from build123d import *

# Parameters (mm, degrees)
F0_W     = 33
F0_H     = 5.5
F1_DEPTH = 2
F2_W     = 33
F2_H     = 2
F3_DEPTH = 33
F4_R     = 3
F5_DEPTH = 2.001


with BuildPart() as f1:
    # F0 (on Top) → F1 (new body)
    with BuildSketch(Plane.XY):
        Rectangle(F0_W, F0_H)
    extrude(amount=F1_DEPTH)

    # F2 (on face) → F3 (join)
    with BuildSketch(Plane.XY.offset(2)):
        with Locations((0, 1.75)):
            Rectangle(F2_W, F2_H)
    extrude(amount=F3_DEPTH)

    # F4 (on face) → F5 (cut, through all)
    with BuildSketch(Plane.XZ.offset(-0.75)):
        with Locations((-9, 17)):
            Circle(F4_R)
        with Locations((9, 17)):
            Circle(F4_R)
    extrude(amount=-F5_DEPTH, mode=Mode.SUBTRACT)


solid = f1.part
Can you work these out from the model? Positions are in its coordinate system, mm. A direction names the side the tool comes from. Round coordinates to 2 decimals unless told otherwise and drop trailing zeros. Write each loop counter-clockwise with the first axis right and the second up, starting at its lowest first coordinate (ties: lowest second). Pieces come first, ordered by that corner, then holes. Notation, with made-up numbers: M -17.75,-36.5 L 40.25,-36.5 A23 cw 40.25,-9.5 Z; hole C 23,-35 d10. An arc over 180 degrees is marked long. Use a Markdown table: item, result.
Item 1: I want a section at D-D (z = 12). List the corners of the cut face in (x, y) for me.
Found:
| item | result |
|---|---|
| outline | M -16.5,0.75 L 16.5,0.75 L 16.5,2.75 L -16.5,2.75 Z |
Item 2: We'd pull the mould along X, two halves only. Please class faces 1 (the face through (-16.5, 1, 13)), 2 (the face through (0, 0, 0)), 3 (the face through (10.384, 1.736, 14.338)): released by +X, released by -X, zero draft, split by the parting line, or undercut.
Found:
| item | result |
|---|---|
| face 1 | released by -X |
| face 2 | zero draft |
| face 3 | undercut |
Item 3: I want a section at B-B (z = 17). List the corners of the cut face in (x, y) for me.
Found:
| item | result |
|---|---|
| outline | M -16.5,0.75 L -12,0.75 L -12,2.75 L -16.5,2.75 Z; M -6,0.75 L 6,0.75 L 6,2.75 L -6,2.75 Z; M 12,0.75 L 16.5,0.75 L 16.5,2.75 L 12,2.75 Z |
Item 4: I want a section at A-A (x = -9). List the corners of the cut face in (y, z) for me.
Found:
| item | result |
|---|---|
| outline | M -2.75,0 L 2.75,0 L 2.75,14 L 0.75,14 L 0.75,2 L -2.75,2 Z; M 0.75,20 L 2.75,20 L 2.75,35 L 0.75,35 Z |
Item 5: If I drill on line 1 along Z through (x, y) = (9, 2); line 2 along Y through (x, z) = (14, 5); line 3 along Z through (x, y) = (1.5, -2.4), over which ranges is the centre line in solid material (lowest first)? Write a range as [from, to].
Found:
| item | result |
|---|---|
| line 1 | z = [0, 14], [20, 35] |
| line 2 | y = [0.75, 2.75] |
| line 3 | z = [0, 2] |
Item 6: Which directions (+Z, -Z, +X, -X, +Y, -Y) give clear straight access to the entire face, cutting with the end or side of a thin tool? Please do faces 4 (the face through (0, 0.75, 18)), 5 (the face through (0, -2.75, 1)).
Found:
| item | result |
|---|---|
| face 4 | +Z, +X, -X, -Y |
| face 5 | +Z, -Z, +X, -X, -Y |
Item 7: I want a section at C-C (x = -12.5). List the corners of the cut face in (y, z) for me, and give its area (3 significant figures).
Found:
| item | result |
|---|---|
| outline | M -2.75,0 L 2.75,0 L 2.75,35 L 0.75,35 L 0.75,2 L -2.75,2 Z |
| area | 77.0 mm2 |
Item 8: For pin 1 Ø1 at (x, y) = (-1.5, -0.5) entering from +Z; pin 2 Ø9.5 at (x, z) = (9, 17) entering from -Y; pin 3 Ø1 at (x, y) = (7, 0.5) entering from +Z, each with a flat end and sliding along its axis, tell me the tip position at first contact or that it passes through.
Found:
| item | result |
|---|---|
| pin 1 | stops at z = 2 |
| pin 2 | stops at y = 0.75 |
| pin 3 | stops at z = 35 |
